```python
from build123d import *

# Parameters (mm, degrees)
F0_R     = 1.6
F0_W     = 5
F0_H     = 5
F0_W_2   = 3
F0_H_2   = 3
F1_DEPTH = 2
F2_DEPTH = 2
F3_R     = 2
F4_R     = 0.5
F5_SIZE  = 0.25


with BuildPart() as f1:
    # F0 (on Top) → F1 (new body)
    with BuildSketch(Plane.XY):
        Polygon((7.5, -7.5), (7.5, 7.5), (1.5, 7.5), (1.5, 4.5), (-1.5, 4.5), (-1.5, 7.5), (-7.5, 7.5), (-7.5, 2.5), (-7.5, -2.5), (-7.5, -7.5), (-1.5, -7.5), (-1.5, -4.5), (1.5, -4.5), (1.5, -7.5), align=None)
        Circle(F0_R, mode=Mode.SUBTRACT)
        with Locations((-10, 0)):
            Rectangle(F0_W, F0_H)
        with Locations((0, 6)):
            Rectangle(F0_W_2, F0_H_2)
        with Locations((0, -6)):
            Rectangle(F0_W_2, F0_H_2)
    extrude(amount=-F1_DEPTH)

    # F0 (on Top) → F2 (join)
    with BuildSketch(Plane.XY):
        with Locations((0, 6)):
            Rectangle(F0_W_2, F0_H_2)
        with Locations((0, -6)):
            Rectangle(F0_W_2, F0_H_2)
    extrude(amount=F2_DEPTH)

    # F3
    f3_edges = [f1.edges().sort_by_distance(p)[0] for p in [
        (-7.5, 2.5, -1),
        (-7.5, -2.5, -1),
    ]]
    fillet(f3_edges, radius=F3_R)

    # F4
    f4_edges = [f1.edges().sort_by_distance(p)[0] for p in [
        (-12.5, 2.5, -1),
        (-12.5, -2.5, -1),
        (-7.5, -7.5, -1),
        (-7.5, 7.5, -1),
        (7.5, 7.5, -1),
        (7.5, -7.5, -1),
        (1.5, 7.5, 1),
        (1.5, 4.5, 1),
        (-1.5, 7.5, 1),
        (-1.5, 4.5, 1),
        (-1.5, -4.5, 1),
        (1.5, -4.5, 1),
        (-1.5, -7.5, 1),
        (1.5, -7.5, 1),
    ]]
    fillet(f4_edges, radius=F4_R)

    # F5
    f5_edges = [f1.edges().sort_by_distance(p)[0] for p in [
        (-7.5, 5.75, -2),
        (-7.353553, 7.353553, -2),
        (-8.085786, 3.085786, -2),
        (0, 7.5, -2),
        (-10.75, 2.5, -2),
        (7.353553, 7.353553, -2),
        (-12.353553, 2.353553, -2),
        (7.5, 0, -2),
        (-12.5, 0, -2),
        (7.353553, -7.353553, -2),
        (-12.353553, -2.353553, -2),
        (0, -7.5, -2),
        (-10.75, -2.5, -2),
        (-7.353553, -7.353553, -2),
        (-8.085786, -3.085786, -2),
        (-7.5, -5.75, -2),
        (-1.6, 0, -2),
    ]]
    chamfer(f5_edges, length=F5_SIZE)


solid = f1.part
```
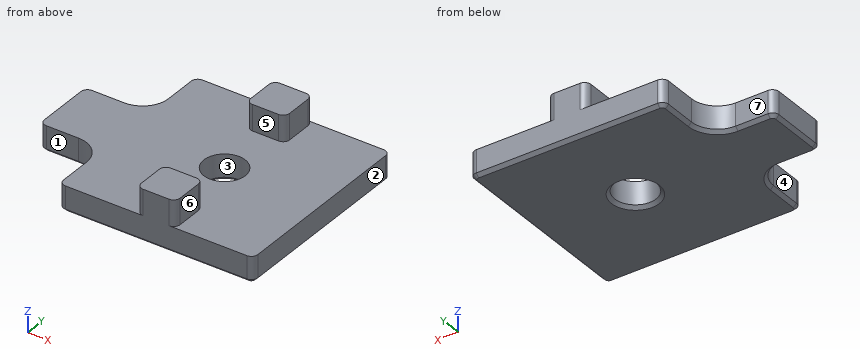
Geometry: final body of the model. Coordinates: model frame, mm. Face numbers are marked on the shaded views. A direction names the side the tool comes from. Round coordinates to 2 decimals unless told otherwise and drop trailing zeros. Order: outer loops, then holes, each group sorted by start corner. A loop starts at its lowest first (then second) coordinate and runs counter-clockwise, first axis right, second up. Notation, with made-up numbers: (13.5, 13.5) -> (66.5, 13.5) arc R33 ccw to (66.5, 44.5) -> close; hole circle Ø9 at (-33.5, 52). An arc over 180 degrees is marked (long way). Write each question's results on one line, items separated by ' | '.
Q1. Ray query, line 1 along Y through (x, z) = (0, -0.9); line 2 along Y through (x, z) = (0.25, 0.65); line 3 along Z through (x, y) = (-6.5, 2.25). Return the intervals inside material, ascending.
Response values:
line 1: -7.5 to -1.6, 1.6 to 7.5 | line 2: -7.5 to -4.5, 4.5 to 7.5 | line 3: -2 to 0
Q2. Pull-direction query (Y, two-part tool) for the marked faces 1, 2 and 3; classes: released by +Y, released by -Y, zero draft, split by the parting line, or undercut.
Response values:
face 1: released by -Y | face 2: zero draft | face 3: undercut
Q3. Section query C-C (x = 0). Output: boundary loops of the cut face in (y, z).
Response values:
outline: (-7.5, -1.75) -> (-7.25, -2) -> (-1.85, -2) -> (-1.6, -1.75) -> (-1.6, 0) -> (-4.5, 0) -> (-4.5, 2) -> (-7.5, 2) -> close; (1.6, -1.75) -> (1.85, -2) -> (7.25, -2) -> (7.5, -1.75) -> (7.5, 2) -> (4.5, 2) -> (4.5, 0) -> (1.6, 0) -> close
Q4. Section query B-B (z = -1). Output: boundary loops of the cut face in (x, y).
Response values:
outline: (-12.5, -2) arc R0.5 ccw to (-12, -2.5) -> (-9.5, -2.5) arc R2 cw to (-7.5, -4.5) -> (-7.5, -7) arc R0.5 ccw to (-7, -7.5) -> (7, -7.5) arc R0.5 ccw to (7.5, -7) -> (7.5, 7) arc R0.5 ccw to (7, 7.5) -> (-7, 7.5) arc R0.5 ccw to (-7.5, 7) -> (-7.5, 4.5) arc R2 cw to (-9.5, 2.5) -> (-12, 2.5) arc R0.5 ccw to (-12.5, 2) -> close; hole circle Ø3.2 at (0, 0)
Q5. Section query D-D (z = 1.5). Output: boundary loops of the cut face in (x, y), and give its area (3 significant figures).
Response values:
outline: (-1.5, -7) arc R0.5 ccw to (-1, -7.5) -> (1, -7.5) arc R0.5 ccw to (1.5, -7) -> (1.5, -5) arc R0.5 ccw to (1, -4.5) -> (-1, -4.5) arc R0.5 ccw to (-1.5, -5) -> close; (-1.5, 5) arc R0.5 ccw to (-1, 4.5) -> (1, 4.5) arc R0.5 ccw to (1.5, 5) -> (1.5, 7) arc R0.5 ccw to (1, 7.5) -> (-1, 7.5) arc R0.5 ccw to (-1.5, 7) -> close | area: 17.6 mm²
Q6. Pin query (flat end, axial travel): pin 1 Ø2 at (x, z) = (-9.5, 0) entering from +Y; pin 2 Ø1.9 at (y, z) = (6, -0.5) entering from -X; pin 3 Ø1.9 at (x, z) = (-11, -0.5) entering from -Y; pin 4 Ø5 at (x, y) = (2.5, 2.5) entering from +Z. Return the tip coordinate at first contact, or that it passes through.
Response values:
pin 1: y = 2.77 | pin 2: x = -7.5 | pin 3: y = -2.5 | pin 4: z = 2
Q7. Section query A-A (y = 0). Output: boundary loops of the cut face in (x, z), and give its area (3 significant figures).
Response values:
outline: (-12.5, -1.75) -> (-12.25, -2) -> (-1.85, -2) -> (-1.6, -1.75) -> (-1.6, 0) -> (-12.5, 0) -> close; (1.6, -1.75) -> (1.85, -2) -> (7.25, -2) -> (7.5, -1.75) -> (7.5, 0) -> (1.6, 0) -> close | area: 33.5 mm²
Q8. Access query for the marked faces 4, 5, 6 and 7. Directions: +Z, -Z, +X, -X, +Y, -Y. A direction counts if a zero-diameter tool reaches every point of the face in a straight line with its end or side. Return the directions, or none.
Response values:
face 4: +Z, -Z, -X, -Y | face 5: +Z, +X, -X | face 6: +Z, +X, +Y, -Y | face 7: +Z, -Z, -X, +Y
